CAD build for the part. Positions are in the model's coordinates, mm. A direction names the side the tool comes from. Round coordinates to 2 decimals unless told otherwise and drop trailing zeros. Write each loop counter-clockwise with the first axis right and the second up, starting at its lowest first coordinate (ties: lowest second). Pieces come first, ordered by that corner, then holes. Notation, with made-up numbers: (-14, -16.5) - (10, -16.5) arc R23 ccw to (10, 9.5) - close; hole circle Ø4 at (-8, 11.5). An arc over 180 degrees is marked (long way). Answer in a Markdown table with one row per item.
```python
from build123d import *

# Parameters (mm, degrees)
F0_R            = 22
F1_DEPTH        = 82
F2_T            = -1.95
F0_R_2          = 28
F3_DEPTH        = 3
F5_R            = 5.05
F6_DEPTH        = 90
F7_R            = 1.55
F8_DEPTH        = 5
F8_COPIES_COUNT = 18
F10_R           = 11
F12_R           = 9.5
F13_DEPTH       = 30


# Not quite as in the source:
# - a pattern or mirror of a feature is missing from the dataset's text; its kind, count and spacing are read off the source's solid


with BuildPart() as f1:
    # F0 (on Top) → F1 (new body)
    with BuildSketch(Plane.XY):
        Circle(F0_R)
    extrude(amount=F1_DEPTH)

    # F2
    f2_openings = [f1.faces().sort_by_distance(p)[0] for p in [
        (0, 0, 0),
    ]]
    offset(amount=F2_T, openings=f2_openings)

    # F0 (on Top) → F3 (join)
    with BuildSketch(Plane.XY):
        Circle(F0_R_2)
        Circle(F0_R, mode=Mode.SUBTRACT)
    extrude(amount=F3_DEPTH)

    # F5 (on Top) → F6 (cut)
    with BuildSketch(Plane.XY):
        Circle(F5_R)
    extrude(amount=F6_DEPTH, mode=Mode.SUBTRACT)

    # F7 (on face) → F8 (cut)
    with BuildSketch(Plane.XY):
        with Locations((-5.3322692402, -24.1057705134)):
            Circle(F7_R)
    f8 = extrude(amount=F8_DEPTH, mode=Mode.SUBTRACT)

    # F8_copies: F8 ×18 about axis
    f8_copies_axis = Axis((0, 0, 0), (0, 0, 1))
    for i in range(1, F8_COPIES_COUNT):
        add(f8.rotate(f8_copies_axis, i * 360 / F8_COPIES_COUNT), mode=Mode.SUBTRACT)

    # F10 (on offset) → F11 (join, up to the next surface of F1)
    with BuildSketch(Plane.XZ.offset(40)):
        with Locations((0, 64.2171450533)):
            Circle(F10_R)
    extrude(until=Until.NEXT, dir=(0, 1, 0))

    # F12 (on face) → F13 (cut)
    with BuildSketch(Plane.XZ.offset(40)):
        with Locations((0, 64.2171450533)):
            Circle(F12_R)
    extrude(amount=-F13_DEPTH, mode=Mode.SUBTRACT)


solid = f1.part
```
Q1. Flat gauge pins, fed straight in: pin 1 (2.5 mm diameter, centred on x = 11.41, y = -21.89, fed in from +Z); pin 2 (4 mm diameter, centred on x = -13.26, y = -20.83, fed in from +Z); pin 3 (6 mm diameter, centred on x = 18, z = 58, fed in from -Y). Where does each tip first touch, or does it go through?
Computed:
| item | result |
|---|---|
| pin 1 | stops at z = 68.43 |
| pin 2 | stops at z = 3 |
| pin 3 | stops at y = -16.09 |
Q2. Saw through at C-C on z = 68.5. List the corners of the cut face in (x, y).
Computed:
| item | result |
|---|---|
| outline | (-10.13, -40) - (-8.48, -40) - (-8.48, -18.17) arc R20.05 cw (long way) to (8.48, -18.17) - (8.48, -40) - (10.13, -40) - (10.13, -19.53) arc R22 ccw (long way) to (-10.13, -19.53) - close |
Q3. Saw through at B-B on z = 34. List the corners of the cut face in (x, y), then the cut area to 3 significant figures.
Computed:
| item | result |
|---|---|
| outline | circle Ø44 at (0, 0); hole circle Ø40.1 at (0, 0) |
| area | 258 mm2 |
Q4. Pull direction X, two halves, no side cores. Call faces 5 (the cylindrical face through (25.865, -10.724, 1.479)), 6 (the cylindrical face through (16.778, -16.077, 1.479)), 7 (the flat face through (19, 8, 0)): released by +X, released by -X, zero draft, split by the parting line, or undercut.
Computed:
| item | result |
|---|---|
| face 5 | split by the parting line |
| face 6 | undercut |
| face 7 | zero draft |
Q5. 3-axis set-ups, long thin cutter, end or side, ignore diameter. For faces 1 (the cylindrical face through (-2.864, 21.813, 41.947)), 2 (the cylindrical face through (-2.61, 19.88, 39.46)), 3 (the cylindrical face through (-2.385, -29.672, 53.479)), 4 (the cylindrical face through (20.81, 15.98, 1.48)): which of +Z, -Z, +X, -X, +Y, -Y reach the whole face in a straight line?
Computed:
| item | result |
|---|---|
| face 1 | none |
| face 2 | -Z |
| face 3 | -Y |
| face 4 | +Z, -Z |
Q6. Drill centre lines: line 1 (Y direction, x = 0, z = 43); line 2 (Z direction, x = 15, y = -3); line 3 (X direction, y = 5, z = 35.5). Where is each one in solid material? Low to high.
Computed:
| item | result |
|---|---|
| line 1 | y = -22 to -20.05, 20.05 to 22 |
| line 2 | z = 80.05 to 82 |
| line 3 | x = -21.42 to -19.42, 19.42 to 21.42 |
Q7. Saw through at A-A on x = 0. List the corners of the cut face in (y, z), then the cut area to 3 significant figures.
Computed:
| item | result |
|---|---|
| outline | (-40, 53.22) - (-22, 53.22) - (-22, 3) - (-28, 3) - (-28, 0) - (-20.05, 0) - (-20.05, 54.72) - (-40, 54.72) - close; (-40, 73.72) - (-20.05, 73.72) - (-20.05, 80.05) - (-5.05, 80.05) - (-5.05, 82) - (-22, 82) - (-22, 75.22) - (-40, 75.22) - close; (5.05, 80.05) - (20.05, 80.05) - (20.05, 0) - (28, 0) - (28, 3) - (22, 3) - (22, 82) - (5.05, 82) - close |
| area | 431 mm2 |
